Can you work these out from the model? Positions are in its coordinate system, mm. A direction names the side the tool comes from. Give positions to 0.01 mm unless a question says otherwise; leave off trailing zeros. Order: outer loops, then holes, each group sorted by start corner. A loop starts at its lowest first (then second) coordinate and runs counter-clockwise, first axis right, second up. Notation, with made-up numbers: M 17.5,18 L 33.5,18 A19 cw 33.5,40 Z; hole C -11.75,79 d2. An arc over 180 degrees is marked long. Write each question's results on one line, items separated by ' | '.
Autodesk Inventor part; units mm, degrees
ref_plane "YZ Plane" through (0, 0, 0) normal (1, 0, 0) x (0, 1, 0)
ref_plane "XZ Plane" through (0, 0, 0) normal (0, 1, 0) x (-1, 0, 0)
ref_plane "XY Plane" through (0, 0, 0) normal (0, 0, 1) x (1, 0, 0)
sketch "Sketch1" plane through (0, 0, 0) normal (0, 1, 0) x (-1, 0, 0)
  line L0 (-9.5, 8.25) -> (9.5, 8.25)
  line L1 (9.5, 8.25) -> (9.5, -8.25)
  line L2 (9.5, -8.25) -> (-9.5, -8.25)
  line L3 (-9.5, -8.25) -> (-9.5, 8.25)
  line L4 (-9.5, 8.25) -> (9.5, -8.25) construction
  line L5 (9.5, 8.25) -> (-9.5, -8.25) construction
  line L6 (-6, 6.75) -> (6, 6.75)
  line L7 (6, 6.75) -> (6, -6.75)
  line L8 (6, -6.75) -> (-6, -6.75)
  line L9 (-6, -6.75) -> (-6, 6.75)
  line L10 (-6, 6.75) -> (6, -6.75) construction
  line L11 (6, 6.75) -> (-6, -6.75) construction
  line L12 (6, -6.75) -> (9.5, -6.75)
  line L13 (-6, -6.75) -> (-9.7082, -6.75)
  line L14 (6, -6.75) -> (6, -8.25)
  line L15 (-6, -6.75) -> (-6, -8.25)
  point P0 (0, 0)
  point P1 (-9.5, -6.75)
  dimension "d0" = 19
  dimension "d1" = 16.5
  dimension "d2" = 12
  dimension "d3" = 1.5
extrude "Extrusion1" add sketch "Sketch1" along normal blind 166 contours L0 L1 L12 L7 L6 L9 L13 L3 | L9 L6 L7 L8 | L8 L14 L2 L15
sketch "Sketch2" plane through (0, 166, 0) normal (0, 1, 0) x (1, 0, 0)
  line L0 (-9.5, -8.25) -> (9.5, -8.25)
  line L1 (9.5, -8.25) -> (0, -8.25)
  line L2 (0, -8.25) -> (0, -0.5)
  line L3 (0, -0.5) -> (9.5, -0.5)
  line L4 (9.5, -0.5) -> (9.5, -8.25)
  circle A0 centre (0, -0.5) radius 5
  point P0 (0, 0)
  dimension "d6" = 7.75
  dimension "d7" = 10
extrude "Extrusion2" add sketch "Sketch2" along normal blind 40 contours A0 L3 L2 | L2 L3 A0
thread "Thread1"
chamfer "Chamfer1" distance 0.5 angle 45 1 edges at (-5, 206, 0.5)
fillet "Fillet1" radius 0.5 8 edges at (9.5, 83, -6.75) (6, 83, -8.25) (9.5, 83, 8.25) (-9.5, 83, 8.25) (-9.5, 83, -6.75) (-6, 83, -6.75) (-6, 83, -8.25) (6, 83, -6.75)
sketch "Sketch3" plane through (-9.5, 0, -6.25) normal (-1, 0, 0) x (0, 0, 1)
  line L0 (14.5, 0) -> (14.5, 166)
  line L1 (14.5, 0) -> (6.75, 0)
  line L2 (6.75, 0) -> (6.75, 206.1896)
  line L3 (6.75, 206.1896) -> (14.5, 206.1896)
  line L4 (14.5, 206.1896) -> (14.5, 0)
  line L5 (6.75, 0) -> (6.75, 20)
  circle A0 centre (6.75, 20) radius 3.5
  point P0 (6.25, 0)
  dimension "d16" = 20
  dimension "d17" = 7
extrude "Extrusion3" cut sketch "Sketch3" against normal through all contours A0 L2 | L2 A0
properties part number "oszlop"
(1) We'd pull the mould along Z, two halves only. Please class faces 3 (the face through (0, 82, -8.25)), 4 (the face through (-9.5, 82, 1)), 5 (the face through (-0.13, 23.47, 0.04)): +Z half, -Z half, draft (parallel to the pull), parting line (faces both ways), or undercut.
Data:
face 3: -Z half | face 4: draft | face 5: undercut
(2) Imagine slicing it at C-C, the plane x = 0. Write out the boundary of the cut face in (y, z), plus the area to 3 significant figures.
Data:
outline: M 0,-8.25 L 166,-8.25 L 166,-4.5 L 205.5,-4.5 L 206,-4 L 206,5 L 205.5,5.5 L 166,5.5 L 166,8.25 L 0,8.25 Z; hole C 20,0.5 d7 | area: 3,100 mm2
(3) Imagine slicing it at A-A, the plane y = 20. Write out the boundary of the cut face in (x, z).
Data:
outline: M -9.5,-6.25 A0.5 ccw -9,-6.75 L -6.5,-6.75 A0.5 cw -6,-7.25 L -6,-7.75 A0.5 ccw -5.5,-8.25 L 5.5,-8.25 A0.5 ccw 6,-7.75 L 6,-7.25 A0.5 cw 6.5,-6.75 L 9,-6.75 A0.5 ccw 9.5,-6.25 L 9.5,-3 L -9.5,-3 Z; M -9.5,4 L 9.5,4 L 9.5,7.75 A0.5 ccw 9,8.25 L -9,8.25 A0.5 ccw -9.5,7.75 Z
(4) Will these pins go through, and if not, where does the flat tip stop? P1, Ø8, axis at x = -6.5, z = 2.5, coming from the -Y side; P2, Ø6, axis at y = 175.5, z = -6.5, coming from the -X side; P3, Ø0.8, axis at x = -7.5, y = 89.5, coming from the -Z side; P4, Ø0.6, axis at y = 79.5, z = -7.5, coming from the -X side.
Data:
P1: stops at y = 0 | P2: stops at x = -3 | P3: stops at z = -6.75 | P4: stops at x = -6
(5) Imagine slicing it at D-D, the plane y = 137. Write out the boundary of the cut face in (x, z), plus the area to 3 significant figures.
Data:
outline: M -9.5,-6.25 A0.5 ccw -9,-6.75 L -6.5,-6.75 A0.5 cw -6,-7.25 L -6,-7.75 A0.5 ccw -5.5,-8.25 L 5.5,-8.25 A0.5 ccw 6,-7.75 L 6,-7.25 A0.5 cw 6.5,-6.75 L 9,-6.75 A0.5 ccw 9.5,-6.25 L 9.5,7.75 A0.5 ccw 9,8.25 L -9,8.25 A0.5 ccw -9.5,7.75 Z | area: 303 mm2
(6) I need wall thicknesses on L1, parallel to Z at x = -0.75, y = 20; L2, parallel to Y at x = 1, z = 0.5; L3, parallel to Y at x = 6.5, z = 0.5. Which ranges of each line are inside material? Lowest first, please. Write a range as from..to.
Data:
L1: z = -8.25..-3, 4..8.25 | L2: y = 0..16.5, 23.5..206 | L3: y = 0..16.5, 23.5..166
(7) Imagine slicing it at B-B, the plane z = 0.5. Write out the boundary of the cut face in (x, y).
Data:
outline: M -9.5,0 L 9.5,0 L 9.5,16.5 L -9.5,16.5 Z; M -9.5,23.5 L 9.5,23.5 L 9.5,166 L 5,166 L 5,205.5 L 4.5,206 L -4.5,206 L -5,205.5 L -5,166 L -9.5,166 Z
(8) For faces 1 (the face through (0, 206, 0)), 2 (the face through (0, 166, 6)), which set-ups out of +Z, -Z, +X, -X, +Y, -Y let a thin tool reach every point of the face, with its end or its side?
Data:
face 1: +Z, -Z, +X, -X, +Y | face 2: +Y
